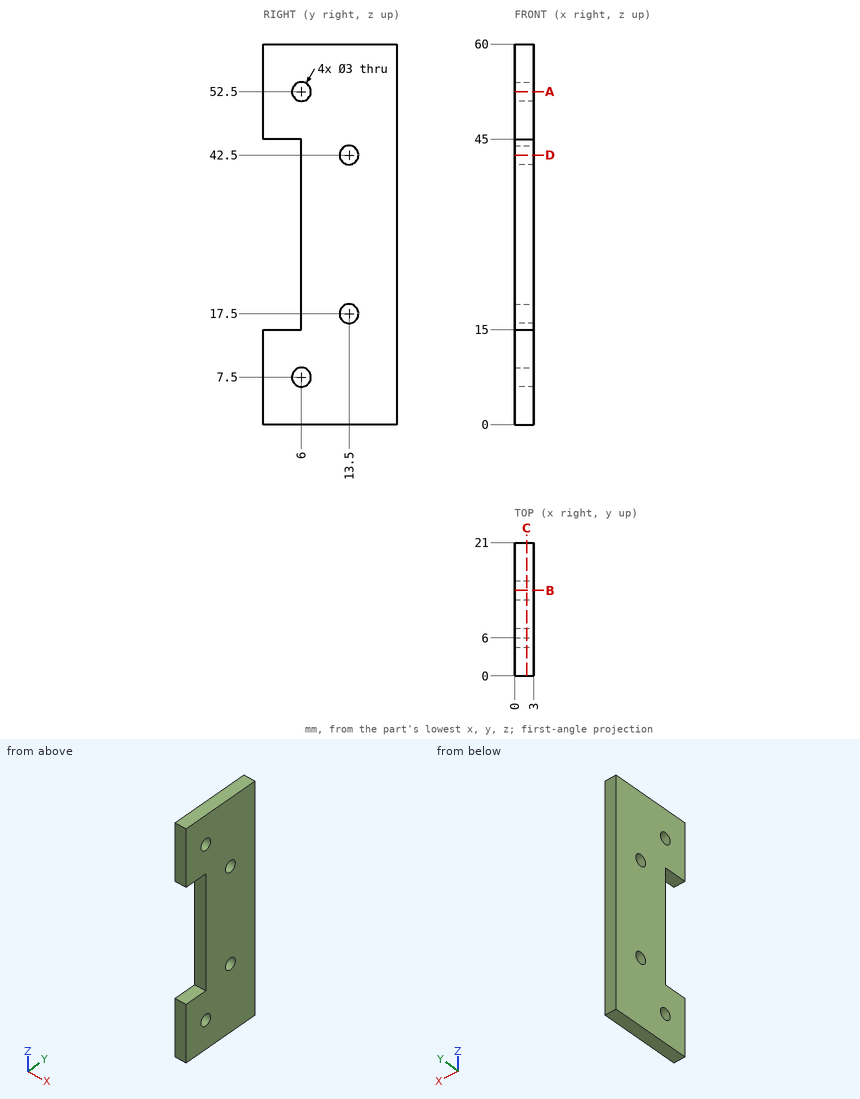
Source: three-view drawing plus pictorial views. Frame: mm from the lowest corner of the part. Give positions to 0.01 mm unless a question says otherwise; leave off trailing zeros. Write each loop counter-clockwise with the first axis right and the second up, starting at its lowest first coordinate (ties: lowest second). Pieces come first, ordered by that corner, then holes. Notation, with made-up numbers: (9.5, 59) -> (58.5, 59) arc R26 ccw to (58.5, 87) -> close; hole circle Ø8 at (71, 20). An arc over 180 degrees is marked (long way). Answer in a Markdown table with one row per item.
(1) Section query A-A on z = 52.5. Return loops of the section in (x, y).
Answers below:
| item | result |
|---|---|
| outline | (0, 0) -> (3, 0) -> (3, 4.5) -> (0, 4.5) -> close; (0, 7.5) -> (3, 7.5) -> (3, 21) -> (0, 21) -> close |
(2) Ray query, line 1 along Y through (x, z) = (1.55, 17.5); line 2 along Z through (x, y) = (2.4, 2.5); line 3 along Y through (x, z) = (2.2, 36). Return the intervals inside material, ascending. Write a range as [from, to].
Answers below:
| item | result |
|---|---|
| line 1 | [6, 12], [15, 21] |
| line 2 | [0, 15], [45, 60] |
| line 3 | [6, 21] |
(3) Pin query (flat end, axial travel): pin 1 (0.9 mm diameter, centred on x = 1.5, y = 3.5, fed in from -Z); pin 2 (1.8 mm diameter, centred on y = 13.5, z = 42.5, fed in from -X). Return the tip coordinate at first contact, or that it passes through.
Answers below:
| item | result |
|---|---|
| pin 1 | z = 0 |
| pin 2 | through |
(4) Section query B-B on y = 13.5. Return loops of the section in (x, z), then the cut area to 3 significant figures.
Answers below:
| item | result |
|---|---|
| outline | (0, 0) -> (3, 0) -> (3, 16) -> (0, 16) -> close; (0, 19) -> (3, 19) -> (3, 41) -> (0, 41) -> close; (0, 44) -> (3, 44) -> (3, 60) -> (0, 60) -> close |
| area | 162 mm^2 |
(5) Section query C-C on x = 1.9. Return loops of the section in (y, z), then the cut area to 3 significant figures.
Answers below:
| item | result |
|---|---|
| outline | (0, 0) -> (21, 0) -> (21, 60) -> (0, 60) -> (0, 45) -> (6, 45) -> (6, 15) -> (0, 15) -> close; hole circle Ø3 at (6, 7.5); hole circle Ø3 at (6, 52.5); hole circle Ø3 at (13.5, 17.5); hole circle Ø3 at (13.5, 42.5) |
| area | 1,050 mm^2 |
(6) Section query D-D on z = 42.5. Return loops of the section in (x, y).
Answers below:
| item | result |
|---|---|
| outline | (0, 6) -> (3, 6) -> (3, 12) -> (0, 12) -> close; (0, 15) -> (3, 15) -> (3, 21) -> (0, 21) -> close |
